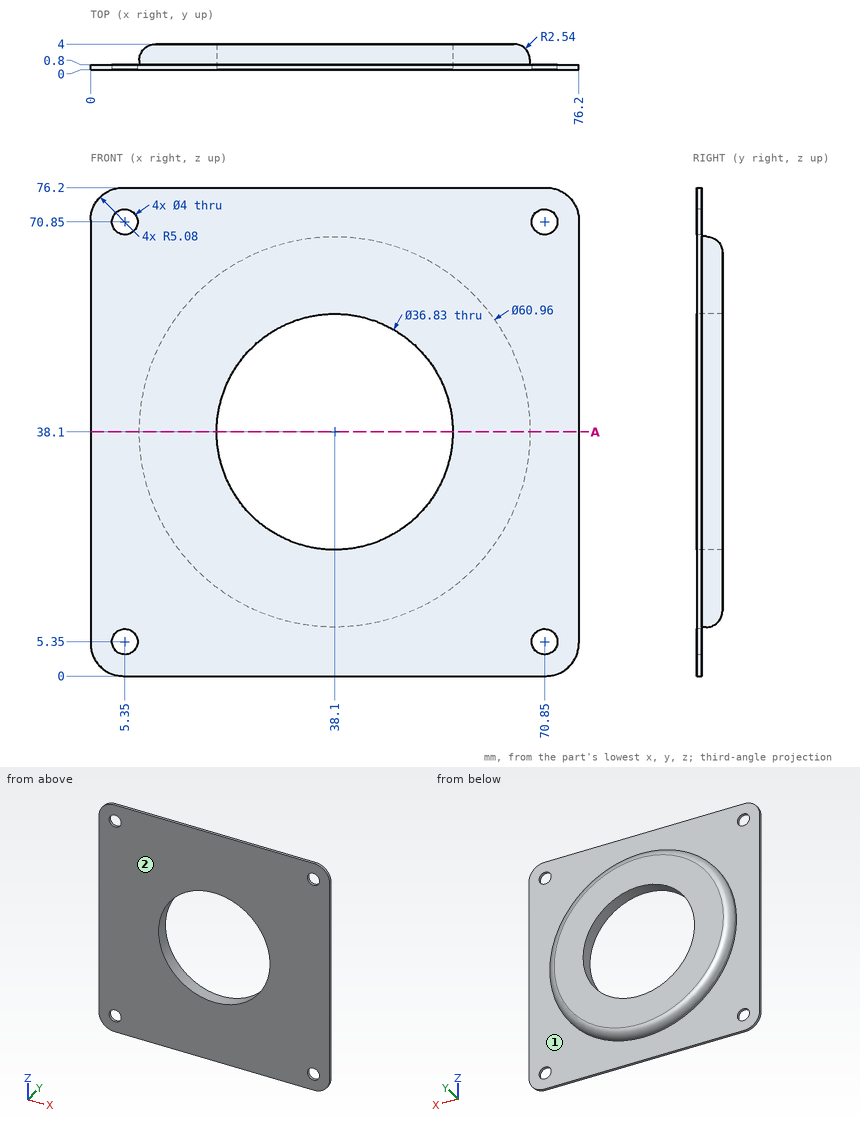
The figure shows three views and two pictorial views of one solid part (mm, origin at its lowest corner). Answer the questions. A direction names the side the tool comes from. Give positions to 0.01 mm unless a question says otherwise; leave off trailing zeros. Loops run counter-clockwise (first coordinate to the right, second up) from the corner with the lowest first, then second, coordinate; pieces in that order, holes last. Notation, with made-up numbers: (55.25, -16.75) - (90.25, -16.75) arc R14 ccw to (90.25, 7.25) - close; hole circle Ø6 at (65, -21). An arc over 180 degrees is marked (long way). Answer in a Markdown table with one row per item.
(1) Section A-A (z = 38.1) is taken. Give the vertices of the cut face in (x, y) (3 decimals), and give its area (3 significant figures).
Results list:
| item | result |
|---|---|
| outline | (0, 0) - (19.685, 0) - (19.685, 4) - (10.16, 4) arc R2.54 ccw to (7.62, 1.46) - (7.62, 0.8) - (0, 0.8) - close; (56.515, 0) - (76.2, 0) - (76.2, 0.8) - (68.58, 0.8) - (68.58, 1.46) arc R2.54 ccw to (66.04, 4) - (56.515, 4) - close |
| area | 106 mm² |
(2) A tool of negligible diameter and unlimited length cuts with its end or side. For the marked faces 1 and 2, from which of +Z, -Z, +X, -X, +Y, -Y can it reach the whole face along a straight path? Write none if from no direction.
Results list:
| item | result |
|---|---|
| face 1 | +Y |
| face 2 | +Z, -Z, +X, -X, -Y |
(3) Consider L1, parallel to Z at x = 70.85, y = 0.45; L2, parallel to Y at x = 16.5, z = 4; L3, parallel to Y at x = 20, z = 16.5. Determine where each line is inside the solid, lowest interval first. Write a range as [from, to].
Results list:
| item | result |
|---|---|
| L1 | z = [0, 3.35], [7.35, 68.85], [72.85, 76.2] |
| L2 | y = [0, 0.8] |
| L3 | y = [0, 3.99] |
(4) Flat-ended cylindrical pins translate along their axes: pin 1 Ø6.5 at (x, z) = (70.85, 5.35) entering from -Y; pin 2 Ø1.5 at (y, z) = (2, 60) entering from +X; pin 3 Ø4.5 at (x, z) = (70.85, 70.85) entering from +Y; pin 4 Ø1 at (y, z) = (1.5, 44.5) entering from +X. Find the tip coordinate at first contact, or state that the pin passes through.
Results list:
| item | result |
|---|---|
| pin 1 | stops at y = 0 |
| pin 2 | stops at x = 59.99 |
| pin 3 | stops at y = 0.8 |
| pin 4 | stops at x = 68 |
